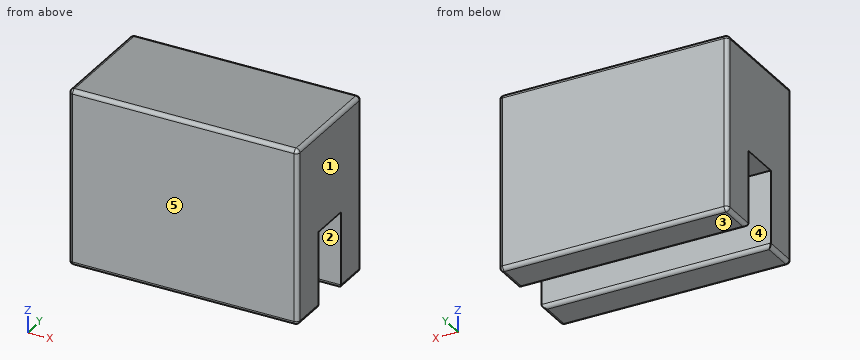
from build123d import *

# Parameters (mm, degrees)
F0_W     = 30
F0_H     = 4.85
F1_DEPTH = 10
F2_W     = 30
F2_H     = 4.85
F2_H_2   = 10.15
F3_DEPTH = 13
F4_R     = 0.5


with BuildPart() as f1:
    # F0 (on Top) → F1 (new body)
    with BuildSketch(Plane.XY):
        with Locations((15, 12.575)):
            Rectangle(F0_W, F0_H)
    extrude(amount=F1_DEPTH)



with BuildPart() as f1b:
    # F0 (on Top) → F1, piece 2 (new body)
    with BuildSketch(Plane.XY):
        with Locations((15, 2.425)):
            Rectangle(F0_W, F0_H)
    extrude(amount=F1_DEPTH)


with BuildPart() as f1_1:
    add(f1.part)

    add(f1b.part)  # F3 merges F1b
    # F2 (on face) → F3 (join)
    with BuildSketch(Plane.XY.offset(10)):
        with Locations((15, 12.575)):
            Rectangle(F2_W, F2_H)
        with Locations((15, 5.075)):
            Rectangle(F2_W, F2_H_2)
    extrude(amount=F3_DEPTH)

    # F4
    f4_edges = [f1_1.edges().sort_by_distance(p)[0] for p in [
        (15, 15, 23),
        (0, 7.5, 23),
        (15, 0, 23),
        (30, 7.5, 23),
        (0, 15, 11.5),
        (30, 15, 11.5),
        (30, 0, 11.5),
        (0, 0, 11.5),
        (0, 2.425, 0),
        (15, 0, 0),
        (30, 2.425, 0),
        (15, 4.85, 0),
        (0, 12.575, 0),
        (30, 12.575, 0),
        (15, 10.15, 0),
        (15, 15, 0),
    ]]
    fillet(f4_edges, radius=F4_R)


solid = f1_1.part
The model under review builds one solid part; all positions refer to its coordinate system, in mm. Face numbers are marked on the shaded views. A direction names the side the tool comes from. Give positions to 0.01 mm unless a question says otherwise; leave off trailing zeros. Write each loop counter-clockwise with the first axis right and the second up, starting at its lowest first coordinate (ties: lowest second). Pieces come first, ordered by that corner, then holes.
1. Tool access review of the marked faces 1 and 2: name each direction out of +Z, -Z, +X, -X, +Y, -Y from which nothing blocks a thin tool from reaching the whole face with its end or side.
2. Wall thickness on L1, parallel to Y at x = 15, z = 3.75; L2, parallel to Z at x = 12.75, y = 5.5; L3, parallel to Z at x = 5, y = 4.75: over which ranges is each line inside the solid? List them lowest first.
3. Draft analysis for pull direction Y (two halves, no side actions). For the marked faces 3, 4 and 5, state which applies: +Y half, -Y half, draft (parallel to the pull), parting line (faces both ways), or undercut.
4. Add section A-A, the plane z = 4.75. Write out the cut boundary in (x, y), plus the area to 3 significant figures.
5. Add section B-B, the plane x = 23.75. Write out the cut boundary in (y, z).
6. Add section C-C, the plane y = 9. Write out the cut boundary in (x, z).
7. For P1, Ø1.6, axis at x = 13.5, y = 7, coming from the -Z side, flat-tipped, find the tip position at first contact; note if it passes through.
Worked answers:
1. face 1: +Z, -Z, +X, +Y, -Y
1. face 2: -Z, +X, -X
2. L1: y = 0 to 4.85, 10.15 to 15
2. L2: z = 10 to 23
2. L3: z = 0.2 to 23
3. face 3: draft
3. face 4: undercut
3. face 5: -Y half
4. outline: (0, 0.5) arc R0.5 ccw to (0.5, 0) - (29.5, 0) arc R0.5 ccw to (30, 0.5) - (30, 4.85) - (0, 4.85) - close; (0, 10.15) - (30, 10.15) - (30, 14.5) arc R0.5 ccw to (29.5, 15) - (0.5, 15) arc R0.5 ccw to (0, 14.5) - close
4. area: 291 mm2
5. outline: (0, 0.5) arc R0.5 ccw to (0.5, 0) - (4.35, 0) arc R0.5 ccw to (4.85, 0.5) - (4.85, 10) - (10.15, 10) - (10.15, 0.5) arc R0.5 ccw to (10.65, 0) - (14.5, 0) arc R0.5 ccw to (15, 0.5) - (15, 22.5) arc R0.5 ccw to (14.5, 23) - (0.5, 23) arc R0.5 ccw to (0, 22.5) - close
6. outline: (0, 10) - (30, 10) - (30, 22.5) arc R0.5 ccw to (29.5, 23) - (0.5, 23) arc R0.5 ccw to (0, 22.5) - close
7. P1: stops at z = 10
